```python
from build123d import *

# Parameters (mm, degrees)
SKETCH1_R           = 2.32
BOSS_EXTRUDE1_DEPTH = 5.33
BOSS_EXTRUDE2_DEPTH = 34.32
SKETCH3_R           = 3.5
SKETCH3_R_2         = 3
BOSS_EXTRUDE3_DEPTH = 2.66
SKETCH4_R           = 2
SKETCH4_R_2         = 1.5
BOSS_EXTRUDE4_DEPTH = 8
BOSS_EXTRUDE5_DEPTH = 12
BOSS_EXTRUDE6_DEPTH = 2
SKETCH7_W           = 10
SKETCH7_H           = 4
BOSS_EXTRUDE7_DEPTH = 5.63


with BuildPart() as part:
    # Sketch1 → Boss-Extrude1 (new body)
    with BuildSketch(Plane(origin=(0, 0, 0), x_dir=(1, 0, 0), z_dir=(0, 1, 0))):
        with BuildLine():
            Line((35.64, -12.5), (-35.64, -12.5))
            ThreePointArc((-35.64, -12.5), (-39.175533906, -11.035533906), (-40.64, -7.5))
            Line((-40.64, -7.5), (-40.64, 7.5))
            ThreePointArc((-40.64, 7.5), (-39.175533906, 11.035533906), (-35.64, 12.5))
            Line((-35.64, 12.5), (35.64, 12.5))
            ThreePointArc((35.64, 12.5), (39.175533906, 11.035533906), (40.64, 7.5))
            Line((40.64, 7.5), (40.64, -7.5))
            ThreePointArc((40.64, -7.5), (39.175533906, -11.035533906), (35.64, -12.5))
        make_face()
        with Locations(Location((-35.95, 0, 0), (0, 0, 270))):
            Circle(SKETCH1_R, mode=Mode.SUBTRACT)
        with Locations(Location((35.95, 0, 0), (0, 0, 270))):
            Circle(SKETCH1_R, mode=Mode.SUBTRACT)
    extrude(amount=BOSS_EXTRUDE1_DEPTH)

    # Sketch2 → Boss-Extrude2 (add)
    with BuildSketch(Plane.XZ):
        with BuildLine():
            Line((23, 16.57), (-23, 16.57))
            ThreePointArc((-23, 16.57), (-28.656854249, 14.226854249), (-31, 8.57))
            Line((-31, 8.57), (-31, -8.57))
            ThreePointArc((-31, -8.57), (-28.656854249, -14.226854249), (-23, -16.57))
            Line((-23, -16.57), (23, -16.57))
            ThreePointArc((23, -16.57), (28.656854249, -14.226854249), (31, -8.57))
            Line((31, -8.57), (31, 8.57))
            ThreePointArc((31, 8.57), (28.656854249, 14.226854249), (23, 16.57))
        make_face()
    extrude(amount=-BOSS_EXTRUDE2_DEPTH)

    # Sketch3 → Boss-Extrude3 (add)
    with BuildSketch(Plane(origin=(0, 34.32, 0), x_dir=(1, 0, 0), z_dir=(0, 1, 0))):
        with Locations(Location((-18.25, 6.35, 0), (0, 0, 270))):
            Circle(SKETCH3_R)
        with Locations(Location((-18.25, -6.35, 0), (0, 0, 270))):
            Circle(SKETCH3_R)
        with Locations(Location((18.25, -6.35, 0), (0, 0, 270))):
            Circle(SKETCH3_R_2)
        with Locations(Location((18.25, 6.35, 0), (0, 0, 270))):
            Circle(SKETCH3_R_2)
    extrude(amount=BOSS_EXTRUDE3_DEPTH)

    # Sketch4 → Boss-Extrude4 (add)
    with BuildSketch(Plane(origin=(0, 36.98, 0), x_dir=(1, 0, 0), z_dir=(0, 1, 0))):
        with Locations(Location((-18.25, 6.35, 0), (0, 0, 270))):
            Circle(SKETCH4_R)
        with Locations(Location((-18.25, -6.35, 0), (0, 0, 270))):
            Circle(SKETCH4_R)
        with Locations(Location((18.25, 6.35, 0), (0, 0, 270))):
            Circle(SKETCH4_R_2)
        with Locations(Location((18.25, -6.35, 0), (0, 0, 270))):
            Circle(SKETCH4_R_2)
    extrude(amount=BOSS_EXTRUDE4_DEPTH)

    # Sketch5 → Boss-Extrude5 (add)
    with BuildSketch(Plane(origin=(0, 34.32, 0), x_dir=(1, 0, 0), z_dir=(0, 1, 0))):
        Polygon((12.25, 1), (-27.5, 1), (-27.5, -1), (12.25, -1), (12.25, -10), (14.25, -10), (14.25, -1), (27.5, -1), (27.5, 1), (14.25, 1), (14.25, 10), (12.25, 10), align=None)
    extrude(amount=BOSS_EXTRUDE5_DEPTH)

    # Sketch6 → Boss-Extrude6 (add)
    with BuildSketch(Plane(origin=(0, 46.32, 0), x_dir=(1, 0, 0), z_dir=(0, 1, 0))):
        with BuildLine():
            Line((-29, 8.57), (-29, -8.57))
            ThreePointArc((-29, -8.57), (-27.242640687, -12.812640687), (-23, -14.57))
            Line((-23, -14.57), (23, -14.57))
            ThreePointArc((23, -14.57), (27.242640687, -12.812640687), (29, -8.57))
            Line((29, -8.57), (29, 8.57))
            ThreePointArc((29, 8.57), (27.242640687, 12.812640687), (23, 14.57))
            Line((23, 14.57), (-23, 14.57))
            ThreePointArc((-23, 14.57), (-27.242640687, 12.812640687), (-29, 8.57))
        make_face()
    extrude(amount=BOSS_EXTRUDE6_DEPTH)

    # Sketch7 → Boss-Extrude7 (add)
    with BuildSketch(Plane(origin=(0, 48.32, 0), x_dir=(1, 0, 0), z_dir=(0, 1, 0))):
        with Locations((-15, 0)):
            Rectangle(SKETCH7_W, SKETCH7_H)
    extrude(amount=BOSS_EXTRUDE7_DEPTH)


solid = part.part
```
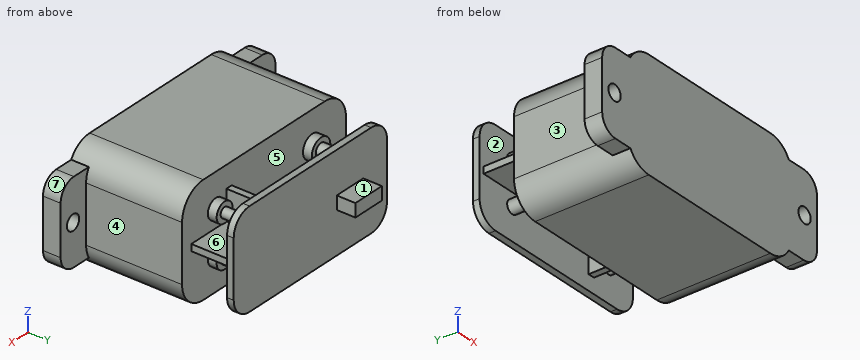
Build history of the part. All positions in model axes, mm. Face numbers are marked on the shaded views. A direction names the side the tool comes from. Round coordinates to 2 decimals unless told otherwise and drop trailing zeros. Loops run counter-clockwise (first coordinate to the right, second up) from the corner with the lowest first, then second, coordinate; pieces in that order, holes last.
Item 1: Pin check, flat tips, straight feed: P1, Ø4, axis at y = 19, z = 5.5, coming from the -X side; P2, Ø4.5, axis at x = -17.5, y = 52.5, coming from the +Z side; P3, Ø6, axis at x = 23, y = 42.5, coming from the +Z side. Stop position of each tip, or through.
Item 2: Saw through at D-D (y = 7). List the corners of the cut face in (x, z), then the cut area to 3 significant figures.
Item 3: Saw through at C-C (x = 18.25). List the corners of the cut face in (y, z), then the cut area to 3 significant figures.
Item 4: Saw through at B-B (y = 35.5). List the corners of the cut face in (x, z), then the cut area to 3 significant figures.
Item 5: Drill centre lines: line 1 along X through (y, z) = (3, 0); line 2 along Y through (x, z) = (23, 10); line 3 along X through (y, z) = (21, -8). Where is each one in solid material? Low to high.
Item 6: Which spindle directions (+Z, -Z, +X, -X, +Y, -Y) get a long thin tool onto all of the face, cutting with end or side? Do the marked faces 1, 2, 3 and 4. Say none if no direction does.
Item 7: Two-plate mould, pull along X, no slides. Class the marked faces 5, 6 and 7: released by +X, released by -X, zero draft, split by the parting line, or undercut.
Item 8: Saw through at A-A (z = 0). List the corners of the cut face in (x, y), then the cut area to 3 significant figures.
Worked answers:
1. P1: stops at x = -31
1. P2: stops at z = 2
1. P3: stops at z = 1
2. outline: (-31, -8.57) arc R8 ccw to (-23, -16.57) - (23, -16.57) arc R8 ccw to (31, -8.57) - (31, 8.57) arc R8 ccw to (23, 16.57) - (-23, 16.57) arc R8 ccw to (-31, 8.57) - close
2. area: 2,000 mm2
3. outline: (0, -16.57) - (34.32, -16.57) - (34.32, -9.35) - (36.98, -9.35) - (36.98, -7.85) - (44.98, -7.85) - (44.98, -4.85) - (36.98, -4.85) - (36.98, -3.35) - (34.32, -3.35) - (34.32, -1) - (46.32, -1) - (46.32, -14.57) - (48.32, -14.57) - (48.32, 14.57) - (46.32, 14.57) - (46.32, 1) - (34.32, 1) - (34.32, 3.35) - (36.98, 3.35) - (36.98, 4.85) - (44.98, 4.85) - (44.98, 7.85) - (36.98, 7.85) - (36.98, 9.35) - (34.32, 9.35) - (34.32, 16.57) - (0, 16.57) - close
3. area: 1,300 mm2
4. outline: (-27.5, -1) - (12.25, -1) - (12.25, -10) - (14.25, -10) - (14.25, -1) - (27.5, -1) - (27.5, 1) - (14.25, 1) - (14.25, 10) - (12.25, 10) - (12.25, 1) - (-27.5, 1) - close; circle Ø7 at (-18.25, -6.35); circle Ø7 at (-18.25, 6.35); circle Ø6 at (18.25, -6.35); circle Ø6 at (18.25, 6.35)
4. area: 280 mm2
5. line 1: x = -40.64 to -38.27, -33.63 to 33.63, 38.27 to 40.64
5. line 2: y = 0 to 34.32, 46.32 to 48.32
5. line 3: x = -31 to 31
6. face 1: +Z, +X, -X, +Y
6. face 2: none
6. face 3: +Z, -Z, -X, +Y
6. face 4: +Z, -Z, +X, +Y
7. face 5: undercut
7. face 6: zero draft
7. face 7: released by +X
8. outline: (-40.64, 0) - (-38.27, 0) - (-38.27, 5.33) - (-40.64, 5.33) - close; (-33.63, 0) - (33.63, 0) - (33.63, 5.33) - (31, 5.33) - (31, 34.32) - (27.5, 34.32) - (27.5, 46.32) - (29, 46.32) - (29, 48.32) - (-10, 48.32) - (-10, 53.95) - (-20, 53.95) - (-20, 48.32) - (-29, 48.32) - (-29, 46.32) - (-27.5, 46.32) - (-27.5, 34.32) - (-31, 34.32) - (-31, 5.33) - (-33.63, 5.33) - close; (38.27, 0) - (40.64, 0) - (40.64, 5.33) - (38.27, 5.33) - close
8. area: 3,010 mm2
